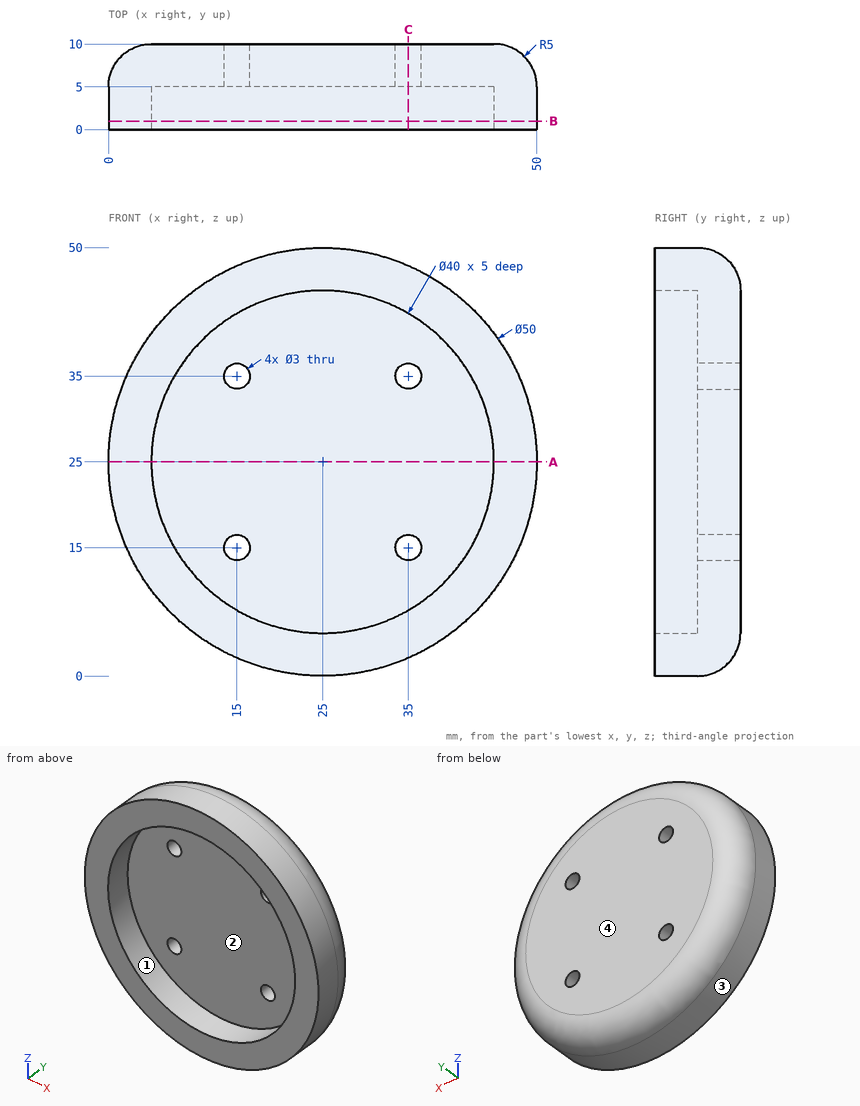
Study the drawing (mm; zero at the part's minimum x, y, z) and answer. Coordinates: 2 decimals unless noted, no trailing zeros. Loops run counter-clockwise (first coordinate to the right, second up) from the corner with the lowest first, then second, coordinate; pieces in that order, holes last. Notation, with made-up numbers: (-6.75, 37.5) -> (20.25, 37.5) arc R17 cw to (20.25, 64.5) -> close; hole circle Ø6 at (85.25, 57.25). An arc over 180 degrees is marked (long way). Answer as CSV lines item,"result".
1) For a pull along X with two mould halves and no side action, classify the marked faces 1, 2, 3 and 4 as released by +X, released by -X, zero draft, split by the parting line, or undercut.
A:
face 1,"undercut"
face 2,"undercut"
face 3,"split by the parting line"
face 4,"zero draft"
2) The part is cut by section A-A (z = 25). Give the vertices of the cut face in (x, y).
A:
outline,"(0, 0) -> (5, 0) -> (5, 5) -> (45, 5) -> (45, 0) -> (50, 0) -> (50, 5) arc R5 ccw to (45, 10) -> (5, 10) arc R5 ccw to (0, 5) -> close"
3) The part is cut by section B-B (y = 1). Give the vertices of the cut face in (x, z).
A:
outline,"circle Ø50 at (25, 25); hole circle Ø40 at (25, 25)"
4) Straight lines are drawn through the part: probe 1 along X at (y, z) = (3.7, 25); probe 2 along X at (y, z) = (8, 35); probe 3 along X at (y, z) = (6.7, 35). For each, find the intervals that lie inside material, in ascending order.
A:
probe 1,"x = 0 to 5, 45 to 50"
probe 2,"x = 3.18 to 13.5, 16.5 to 33.5, 36.5 to 46.82"
probe 3,"x = 2.41 to 13.5, 16.5 to 33.5, 36.5 to 47.59"
5) The part is cut by section C-C (x = 35). State how many separate pieces and enclosed holes the cut face has, and give its area (3 significant figures).
A:
separate pieces,"3"
enclosed holes,"0"
area,"243 mm²"
6) Flat-ended cylindrical pins translate along their axes: pin 1 (3.5 mm diameter, centred on x = 15, z = 35, fed in from -Y); pin 2 (4 mm diameter, centred on x = 43.5, y = 5.5, fed in from -Z); pin 3 (3 mm diameter, centred on y = 3, z = 42, fed in from -X). Find the tip coordinate at first contact, or state that the pin passes through.
A:
pin 1,"stops at y = 5"
pin 2,"stops at z = 6.24"
pin 3,"stops at x = 5.38"
